from build123d import *

# Parameters (mm, degrees)
SKETCH1_R               = 2.4
BOSS_EXTRUDE1_DEPTH     = 2.2
BOSS_EXTRUDE1_TAPER     = 10
SKETCH2_R               = 1.6
BOSS_EXTRUDE2_DEPTH     = 3.5
CUT_EXTRUDE1_DEPTH      = 12.802330327
CUT_EXTRUDE1_DEPTH_BACK = 12.802330327
SKETCH4_R               = 1.26


with BuildPart() as part:
    # Sketch1 → Boss-Extrude1 (new body)
    with BuildSketch(Plane(origin=(0, 0, 0), x_dir=(1, 0, 0), z_dir=(0, 1, 0))):
        Circle(SKETCH1_R)
    extrude(amount=BOSS_EXTRUDE1_DEPTH, taper=BOSS_EXTRUDE1_TAPER)

    # Sketch2 → Boss-Extrude2 (add)
    with BuildSketch(Plane.XZ):
        with BuildLine():
            Line((-5.95, -2.5), (-5.95, 2.5))
            ThreePointArc((-5.95, 2.5), (0, 8.45), (5.95, 2.5))
            Line((5.95, 2.5), (5.95, -2.5))
            ThreePointArc((5.95, -2.5), (0, -8.45), (-5.95, -2.5))
        make_face()
        with Locations(Location((0, -5, 0), (0, 0, 270))):
            Circle(SKETCH2_R, mode=Mode.SUBTRACT)
        with Locations(Location((0, 5, 0), (0, 0, 270))):
            Circle(SKETCH2_R, mode=Mode.SUBTRACT)
    extrude(amount=BOSS_EXTRUDE2_DEPTH)

    # Sketch4 → Cut-Extrude1 (cut, two sides: drawn at the far end of the back side and taken through both)
    with BuildSketch(Plane.XZ.offset(3.5).offset(-CUT_EXTRUDE1_DEPTH_BACK)):
        with Locations(Location((0, 0, 0), (0, 0, 270))):
            Circle(SKETCH4_R)
    extrude(amount=CUT_EXTRUDE1_DEPTH + CUT_EXTRUDE1_DEPTH_BACK, mode=Mode.SUBTRACT)


solid = part.part
Here's how the part is built. I have some questions about the finished solid (model axes, mm). Give positions to 0.01 mm unless a question says otherwise; leave off trailing zeros. Loops run counter-clockwise (first coordinate to the right, second up) from the corner with the lowest first, then second, coordinate; pieces in that order, holes last. Notation, with made-up numbers: (-26, 69) -> (0, 69) arc R16 ccw to (0, 78) -> close; hole circle Ø6 at (40.25, 66.5). An arc over 180 degrees is marked (long way). One line per item, written item: value.
Q1. We'd pull the mould along X, two halves only. Please class faces 1 (the face through (5.95, -2, 0)), 2 (the face through (-0.97, -1.73, 6.27)), 3 (the face through (0.13, -1.73, -8.45)): pulls with the +X half, pulls with the -X half, needs draft (parallel to the pull), parting line crosses it, or undercut.
Answers follow:
face 1: pulls with the +X half
face 2: undercut
face 3: parting line crosses it
Q2. Suppose I cut it at C-C on z = 3.75. Please give me the cut outline in (x, y), then the cut area to 3 significant figures.
Answers follow:
outline: (-5.82, -3.5) -> (-1, -3.5) -> (-1, 0) -> (-5.82, 0) -> close; (1, -3.5) -> (5.82, -3.5) -> (5.82, 0) -> (1, 0) -> close
area: 33.7 mm^2
Q3. Suppose I cut it at A-A on y = -1.85. Please give me the cut outline in (x, z), then the cut area to 3 significant figures.
Answers follow:
outline: (-5.95, -2.5) arc R5.95 ccw to (5.95, -2.5) -> (5.95, 2.5) arc R5.95 ccw to (-5.95, 2.5) -> close; hole circle Ø3.2 at (0, -5); hole circle Ø3.2 at (0, 5); hole circle Ø2.52 at (0, 0)
area: 150 mm^2
Q4. Suppose I cut it at D-D on z = -5. Please give me the cut outline in (x, y), then the cut area to 3 significant figures.
Answers follow:
outline: (-5.4, -3.5) -> (-1.6, -3.5) -> (-1.6, 0) -> (-5.4, 0) -> close; (1.6, -3.5) -> (5.4, -3.5) -> (5.4, 0) -> (1.6, 0) -> close
area: 26.6 mm^2
Q5. Suppose I cut it at B-B on x = 0. Please give me the cut outline in (y, z), then the cut area to 3 significant figures.
Answers follow:
outline: (-3.5, -8.45) -> (0, -8.45) -> (0, -6.6) -> (-3.5, -6.6) -> close; (-3.5, -3.4) -> (0, -3.4) -> (0, -2.4) -> (2.2, -2.01) -> (2.2, -1.26) -> (-3.5, -1.26) -> close; (-3.5, 1.26) -> (2.2, 1.26) -> (2.2, 2.01) -> (0, 2.4) -> (0, 3.4) -> (-3.5, 3.4) -> close; (-3.5, 6.6) -> (0, 6.6) -> (0, 8.45) -> (-3.5, 8.45) -> close
area: 32.1 mm^2
Q6. If I drill on line 1 along X through (y, z) = (-0.75, 0); line 2 along Y through (x, z) = (5.5, 2); line 3 along X through (y, z) = (-2.35, 5), over which ranges is the centre line in solid material (lowest first)?
Answers follow:
line 1: -5.95 to -1.26, 1.26 to 5.95
line 2: -3.5 to 0
line 3: -5.4 to -1.6, 1.6 to 5.4
